Design review of the part built by this model. Coordinates are the model's own, in mm. Coordinates: 2 decimals unless noted, no trailing zeros. Order: outer loops, then holes, each group sorted by start corner. A loop starts at its lowest first (then second) coordinate and runs counter-clockwise, first axis right, second up. Notation, with made-up numbers: (18, 62) - (32, 62) arc R7 ccw to (32, 70) - close; hole circle Ø11 at (-10, 22.5). An arc over 180 degrees is marked (long way). Write each question's results on one line, items separated by ' | '. Start each with the question number.
```python
from build123d import *

# Parameters (mm, degrees)
BOSS_EXTRU_1_START      = -4
BOSS_EXTRU_1_DEPTH      = 2
ESQUISSE2_R             = 1.5
ENL_V_MAT_EXTRU_1_DEPTH = 2


with BuildPart() as part:
    # Esquisse1 → Boss.-Extru.1 (new body)
    with BuildSketch(Plane.XY.offset(BOSS_EXTRU_1_START)):
        with BuildLine():
            Line((-20.180030535, -16.314431829), (0.97983118, -7.299984969))
            ThreePointArc((0.97983118, -7.299984969), (2.40785155, -4.327503968), (-0.353745657, -2.52515374))
            ThreePointArc((-0.353745657, -2.52515374), (-0.672496032, -2.59214845), (-0.97983118, -2.700015031))
            Line((-0.97983118, -2.700015031), (-6.059542219, -4.86405494))
            Line((-6.059542219, -4.86405494), (-22.139692896, -11.714461891))
            ThreePointArc((-22.139692896, -11.714461891), (-23.459846684, -14.994278041), (-20.180030535, -16.314431829))
        make_face()
    extrude(amount=BOSS_EXTRU_1_DEPTH)

    # Esquisse2 → Enlèv. mat.-Extru.1 (cut)
    with BuildSketch(Plane.XY.offset(-2)):
        with Locations((-21.159861715, -14.01444686)):
            Circle(ESQUISSE2_R)
        with Locations((0, -5)):
            Circle(ESQUISSE2_R)
    extrude(amount=-ENL_V_MAT_EXTRU_1_DEPTH, mode=Mode.SUBTRACT)


solid = part.part
```
(1) Take a section at A-A (y = -15.25). State the section outline as (x, z) points.
(2) Take a section at D-D (x = -18). State the section outline as (y, z) points.
(3) To check wall thickness, follow line 1 along Y through (x, z) = (0, -2.45); line 2 along X through (y, z) = (-4.5, -2.2); line 3 along X through (y, z) = (-5.75, -2.7). State the ranges of each line that lie inside material, in increasing order. Write a range as [from, to].
(4) Mouldability with a two-part tool opening along Y and no side actions: class faces 1 (the face through (-0.195, -3.513, -2.986)), 2 (the face through (-11, -9, -4)), 3 (the face through (-23.481, -14.943, -3.014)), 4 (the face through (-19.73, -13.56, -2.99)) as +Y half, -Y half, draft (parallel to the pull), parting line (faces both ways), or undercut.
(5) Take a section at B-B (x = 0). State the section outline as (y, z) points.
(6) Take a section at C-C (z = -2.3). State the section outline as (x, y) points, plus the area to 3 significant figures.
Worked out:
1) outline: (-23.33, -4) - (-22.01, -4) - (-22.01, -2) - (-23.33, -2) - close; (-20.31, -4) - (-17.68, -4) - (-17.68, -2) - (-20.31, -2) - close
2) outline: (-15.39, -4) - (-9.95, -4) - (-9.95, -2) - (-15.39, -2) - close
3) line 1: [-7.72, -6.5], [-3.5, -2.5] | line 2: [-5.2, -1.41], [1.41, 2.45] | line 3: [-8.14, -1.3], [1.3, 2.38]
4) face 1: undercut | face 2: draft | face 3: parting line | face 4: undercut
5) outline: (-7.72, -4) - (-6.5, -4) - (-6.5, -2) - (-7.72, -2) - close; (-3.5, -4) - (-2.5, -4) - (-2.5, -2) - (-3.5, -2) - close
6) outline: (-22.14, -11.71) arc R2.5 ccw to (-20.18, -16.31) - (0.98, -7.3) arc R2.5 ccw to (-0.98, -2.7) - close; hole circle Ø3 at (-21.16, -14.01); hole circle Ø3 at (0, -5) | area: 120 mm^2
